```python
from build123d import *

# Parameters (mm, degrees)
SKETCH_1_R          = 2
EXTRUDE_1_DEPTH     = 32.5
CUT_EXTRUDE_START   = -1
SKETCH_2_R          = 2
SKETCH_2_R_2        = 0.75
CUT_EXTRUDE_1_DEPTH = 5
FILLET_1_R          = 0.5


with BuildPart() as part:
    # ｽｹｯﾁ1 → ﾎﾞｽ - 押し出し1 (new body)
    with BuildSketch(Plane(origin=(0, 0, 0), x_dir=(1, 0, 0), z_dir=(0, 1, 0))):
        Circle(SKETCH_1_R)
    extrude(amount=EXTRUDE_1_DEPTH)

    # ｽｹｯﾁ2 → ｶｯﾄ - 押し出し1 (cut)
    with BuildSketch(Plane.XZ.offset(CUT_EXTRUDE_START)):
        Circle(SKETCH_2_R)
        Circle(SKETCH_2_R_2, mode=Mode.SUBTRACT)
    extrude(amount=-CUT_EXTRUDE_1_DEPTH, mode=Mode.SUBTRACT)

    # ﾌｨﾚｯﾄ1
    fillet_1_edges = [part.edges().sort_by_distance(p)[0] for p in [
        (-2, 32.5, 0),
    ]]
    fillet(fillet_1_edges, radius=FILLET_1_R)


solid = part.part
```
Part model, mm, in its own coordinate system. A direction names the side the tool comes from. Give positions to 0.01 mm unless a question says otherwise; leave off trailing zeros. Write each loop counter-clockwise with the first axis right and the second up, starting at its lowest first coordinate (ties: lowest second). Pieces come first, ordered by that corner, then holes. Notation, with made-up numbers: M 62,-19 L 108,-19 A37 ccw 108,20 Z; hole C 1,48.25 d5. An arc over 180 degrees is marked long. Use CSV: the item, a comma, the result in double quotes.
Item 1: Slice it at D-D on y = 3.5. Write the cut outline in (x, z).
Taken from the geometry:
outline,"C 0,0 d1.5"
Item 2: Pin check, flat tips, straight feed: P1, Ø1, axis at x = -1, y = 20, coming from the -Z side; P2, Ø1.5, axis at y = 23.5, z = -1.5, coming from the +X side; P3, Ø1.5, axis at y = 21, z = -1, coming from the -X side. Stop position of each tip, or through.
Taken from the geometry:
P1,"stops at z = -1.94"
P2,"stops at x = 1.85"
P3,"stops at x = -1.98"
Item 3: Drill centre lines: probe 1 along Y at (x, z) = (0.9, 1.3); probe 2 along X at (y, z) = (20, 0.1); probe 3 along Z at (x, y) = (0.85, 22.5). Where is each one in solid material? Low to high.
Taken from the geometry:
probe 1,"y = 0 to 1, 6 to 32.49"
probe 2,"x = -2 to 2"
probe 3,"z = -1.81 to 1.81"
Item 4: Slice it at A-A on z = 0. Write the cut outline in (x, y).
Taken from the geometry:
outline,"M -2,0 L 2,0 L 2,1 L 0.75,1 L 0.75,6 L 2,6 L 2,32 A0.5 ccw 1.5,32.5 L -1.5,32.5 A0.5 ccw -2,32 L -2,6 L -0.75,6 L -0.75,1 L -2,1 Z"
Item 5: Slice it at C-C on y = 30. Write the cut outline in (x, z).
Taken from the geometry:
outline,"C 0,0 d4"
Item 6: Pull direction Y, two halves, no side cores. Call faces 1 (the face through (1, 6, 0)), 2 (the face through (0, 0, 0)), 3 (the face through (-0.434, 0.493, 1.952)), 4 (the face through (-0.75, 3.46, 0.03)): +Y half, -Y half, draft (parallel to the pull), parting line (faces both ways), or undercut.
Taken from the geometry:
face 1,"undercut"
face 2,"-Y half"
face 3,"draft"
face 4,"undercut"
Item 7: Which spindle directions (+Z, -Z, +X, -X, +Y, -Y) get a long thin tool onto all of the face, cutting with end or side? Do faces 5 (the face through (0, 32.5, 0)), 6 (the face through (1, 1, 0)). Say none if no direction does.
Taken from the geometry:
face 5,"+Z, -Z, +X, -X, +Y"
face 6,"none"
Item 8: Slice it at B-B on x = 0. Write the cut outline in (y, z).
Taken from the geometry:
outline,"M 0,-2 L 1,-2 L 1,-0.75 L 6,-0.75 L 6,-2 L 32,-2 A0.5 ccw 32.5,-1.5 L 32.5,1.5 A0.5 ccw 32,2 L 6,2 L 6,0.75 L 1,0.75 L 1,2 L 0,2 Z"
